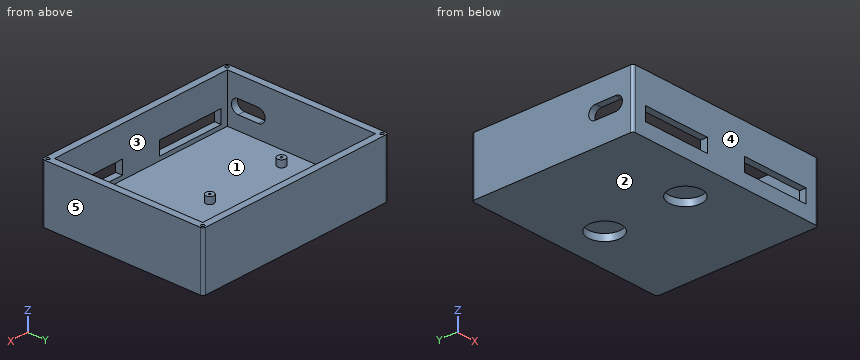
Autodesk Fusion 360 part; units mm, degrees
sketch "スケッチ6" plane through (0, 0, 0) normal (0, 0, 1) x (1, 0, 0)
  line L0 (75, -45) -> (-75, -45)
  line L1 (-75, -45) -> (-75, 75)
  line L2 (-75, 75) -> (75, 75)
  line L3 (75, 75) -> (75, -45)
  line L4 (-200, 0) -> (160, 0)
  dimension "d22" = 150
  dimension "d110" = 75
  dimension "d111" = 45
extrude "押し出し4" add sketch "スケッチ6" along normal blind 42
sketch "スケッチ7" plane through (0, 0, 42) normal (0, 0, 1) x (-1, 0, 0)
  line L0 (-75, -75) -> (75, -75)
  line L1 (75, -75) -> (75, 45)
  line L2 (75, 45) -> (-75, 45)
  line L3 (-75, 45) -> (-75, -75)
  line L4 (70, -70) -> (-70, -70)
  line L5 (-70, -70) -> (-70, 40)
  line L6 (-70, 40) -> (70, 40)
  line L7 (70, 40) -> (70, -70)
  dimension "d26" = 5
  dimension "d27" = 5
extrude "押し出し5" cut sketch "スケッチ7" against normal blind 35 contours L4 L5 L6 L7
sketch "スケッチ8" plane through (0, 0, 7) normal (0, 0, 1) x (-1, 0, 0)
  line L0 (70, 40) -> (-70, 40)
  line L1 (-70, 40) -> (-70, -70)
  line L2 (-70, -70) -> (70, -70)
  line L3 (70, -70) -> (70, 40)
  circle A0 centre (56.5, -61.5) radius 3
  circle A1 centre (-1.5, -61.5) radius 3
  circle A2 centre (56.5, -12.5) radius 3
  circle A3 centre (-1.5, -12.5) radius 3
  dimension "d32" = 6
  dimension "d35" = 6
  dimension "d37" = 58
  dimension "d41" = 6
  dimension "d42" = 6
extrude "押し出し6" add sketch "スケッチ8" along normal blind 5 contours A0 | A1 | A2 | A3
sketch "スケッチ9" plane through (0, 0, 12) normal (0, 0, 1) x (-1, 0, 0)
  circle A0 centre (56.5, -61.5) radius 3
  line L0 (56.5, -61.5) -> (53.5, -61.5)
  line L1 (56.5, -61.5) -> (56.5, -64.5)
hole "穴1" at (-56.5, 61.5, 12) direction (0, 0, -1) diameter 1.623 depth 10 tip angle 118
sketch "スケッチ10" plane through (0, 0, 12) normal (0, 0, 1) x (-1, 0, 0)
  circle A0 centre (-1.5, -61.5) radius 3
  line L0 (-1.5, -61.5) -> (-3.2909, -61.5)
  line L1 (-3.2909, -61.5) -> (-1.5, -61.5)
  line L2 (-1.5, -61.5) -> (-1.5, -64)
hole "穴2" at (1.5, 61.5, 12) direction (0, 0, -1) diameter 1.623 depth 10 tip angle 118
sketch "スケッチ11" plane through (0, 0, 12) normal (0, 0, 1) x (-1, 0, 0)
  circle A0 centre (-1.5, -12.5) radius 3
  line L0 (-1.5, -12.5) -> (-4.5, -12.5)
  line L1 (-1.5, -12.5) -> (-1.5, -15.5)
hole "穴3" at (1.5, 12.5, 12) direction (0, 0, -1) diameter 1.623 depth 10 tip angle 118
sketch "スケッチ12" plane through (0, 0, 12) normal (0, 0, 1) x (-1, 0, 0)
  circle A0 centre (56.5, -12.5) radius 3
  line L0 (56.5, -12.5) -> (53.5, -12.5)
  line L1 (56.5, -12.5) -> (56.5, -15.5)
hole "穴4" at (-56.5, 12.5, 12) direction (0, 0, -1) diameter 1.623 depth 10 tip angle 118
sketch "スケッチ13" plane through (-75, 0, 0) normal (-1, 0, 0) x (0, -1, 0)
  line L0 (-75, 0) -> (45, 0)
  line L1 (45, 0) -> (45, 42)
  line L2 (45, 42) -> (-75, 42)
  line L3 (-75, 42) -> (-75, 0)
  line L4 (17, 27) -> (32, 27)
  line L5 (32, 17) -> (25.3423, 17)
  arc A0 (32, 17) -> (32, 27) centre (32, 22) ccw
  line L6 (25.3423, 17) -> (17, 17)
  arc A1 (17, 27) -> (17, 17) centre (17, 22) ccw
  dimension "d55" = 15
  dimension "d56" = 10
extrude "押し出し7" cut sketch "スケッチ13" against normal blind 10 contours L4 L5 A0 L6 A1
sketch "スケッチ15" plane through (0, -45, 0) normal (0, -1, 0) x (1, 0, 0)
  line L0 (-75, 0) -> (75, 0)
  line L1 (75, 0) -> (75, 42)
  line L2 (75, 42) -> (-75, 42)
  line L3 (-75, 42) -> (-75, 0)
  line L4 (-15, 10) -> (-65, 10)
  line L5 (-65, 10) -> (-65, 20)
  line L6 (-65, 20) -> (-15, 20)
  line L7 (-15, 20) -> (-15, 10)
  line L8 (15, 20) -> (65, 20)
  line L9 (65, 20) -> (65, 10)
  line L10 (65, 10) -> (15, 10)
  line L11 (15, 10) -> (15, 20)
extrude "押し出し8" cut sketch "スケッチ15" against normal blind 5 contours L4 L5 L6 L7 | L8 L9 L10 L11
sketch "スケッチ16" plane through (0, 0, 42) normal (0, 0, 1) x (-1, 0, 0)
  line L0 (-70, -70) -> (-70, 40)
  line L1 (-70, 40) -> (70, 40)
  line L2 (70, 40) -> (70, -70)
  line L3 (70, -70) -> (-70, -70)
  line L4 (-75, -75) -> (75, -75)
  line L5 (75, -75) -> (75, 45)
  line L6 (75, 45) -> (-75, 45)
  line L7 (-75, 45) -> (-75, -75)
  circle A0 centre (72.5, -72.5) radius 1.5
  circle A1 centre (-72.5, -72.5) radius 1.5
  circle A2 centre (72.5, 72.5) radius 1.5
  circle A3 centre (-72.5, 72.5) radius 1.5
  dimension "d96" = 3
  dimension "d97" = 2.5
  dimension "d98" = 2.5
hole "穴5" at (-72.5, 72.5, 42) at (-72.5, -72.5, 42) at (72.5, 72.5, 42) at (72.5, -72.5, 42) direction (0, 0, -1) diameter 2.529 depth 10 tip angle 118
sketch "スケッチ17" plane through (0, 0, 0) normal (0, 0, 1) x (1, 0, 0)
  circle A0 centre (0, 45) radius 11.95
  circle A1 centre (0, -15) radius 11.95
  line L0 (-75, 75) -> (75, 75)
  line L1 (75, -45) -> (-75, -45)
  dimension "d102" = 23.9
  dimension "d103" = 23.9
  dimension "d104" = 30
  dimension "d105" = 30
extrude "押し出し9" cut sketch "スケッチ17" along normal blind 5
fillet "フィレット1" radius 2 4 edges at (75, -45, 21) (-75, -45, 21) (75, 75, 21) (-75, 75, 21)
sketch "スケッチ18" plane through (0, 0, 42) normal (0, 0, 1) x (-1, 0, 0)
  arc A0 (73, -75) -> (75, -73) centre (73, -73) ccw
  line L0 (75, -73) -> (75, 43)
  arc A1 (75, 43) -> (73, 45) centre (73, 43) ccw
  line L1 (73, 45) -> (-73, 45)
  arc A2 (-73, 45) -> (-75, 43) centre (-73, 43) ccw
  line L2 (-75, 43) -> (-75, -73)
  arc A3 (-75, -73) -> (-73, -75) centre (-73, -73) ccw
  line L3 (-73, -75) -> (73, -75)
  circle A4 centre (-72.5, -72.5) radius 1.2645
  circle A5 centre (72.5, -72.5) radius 1.2645
  line L4 (-70, -70) -> (-70, 40)
  line L5 (-70, 40) -> (70, 40)
  line L6 (70, 40) -> (70, -70)
  line L7 (70, -70) -> (-70, -70)
  circle A6 centre (72.5, 42.5) radius 1
  circle A7 centre (-72.5, 42.5) radius 1
  dimension "d112" = 2
  dimension "d113" = 2.5
  dimension "d114" = 2.5
  dimension "d115" = 2
  dimension "d116" = 2.5
  dimension "d117" = 2.5
hole "穴6" at (-72.5, -42.5, 42) at (72.5, -42.5, 42) direction (0, 0, -1) diameter 2.529 depth 10 tip angle 118
equation "d111 = 75 mm - 30 mm"
Could you check a few things on this model? Use its own coordinates, in mm. Face numbers are marked on the shaded views. A direction names the side the tool comes from. Coordinates: 2 decimals unless noted, no trailing zeros. Loops run counter-clockwise (first coordinate to the right, second up) from the corner with the lowest first, then second, coordinate; pieces in that order, holes last. Notation, with made-up numbers: (62.5, 87) -> (86.5, 87) arc R17 ccw to (86.5, 106) -> close; hole circle Ø4 at (87, 66.25). An arc over 180 degrees is marked (long way). Answer in a Markdown table with one row per item.
(1) Thinking about a two-plate mould opening in Y: for the marked faces 3, 4 and 5, which applies, released by +Y, released by -Y, zero draft, split by the parting line, or undercut?
Results found:
| item | result |
|---|---|
| face 3 | undercut |
| face 4 | released by -Y |
| face 5 | zero draft |
(2) Imagine slicing it at D-D (y = -20). List the corners of the cut face in (x, z) for me, plus the area to 3 significant figures.
Results found:
| item | result |
|---|---|
| outline | (-75, 0) -> (-10.85, 0) -> (-10.85, 5) -> (10.85, 5) -> (10.85, 0) -> (75, 0) -> (75, 42) -> (70, 42) -> (70, 7) -> (-70, 7) -> (-70, 17) -> (-75, 17) -> close; (-75, 27) -> (-70, 27) -> (-70, 42) -> (-75, 42) -> close |
| area | 1,240 mm^2 |
(3) For the marked faces 1 and 2, which set-ups out of +Z, -Z, +X, -X, +Y, -Y let a thin tool reach every point of the face, with its end or its side?
Results found:
| item | result |
|---|---|
| face 1 | +Z |
| face 2 | -Z, +X, -X, +Y, -Y |
(4) Imagine slicing it at C-C (z = 22). List the corners of the cut face in (x, y) for me.
Results found:
| item | result |
|---|---|
| outline | (-75, -43) arc R2 ccw to (-73, -45) -> (73, -45) arc R2 ccw to (75, -43) -> (75, 73) arc R2 ccw to (73, 75) -> (-73, 75) arc R2 ccw to (-75, 73) -> (-75, -12) -> (-70, -12) -> (-70, 70) -> (70, 70) -> (70, -40) -> (-70, -40) -> (-70, -37) -> (-75, -37) -> close |
(5) Imagine slicing it at B-B (y = 23). List the corners of the cut face in (x, z) for me, plus the area to 3 significant figures.
Results found:
| item | result |
|---|---|
| outline | (-75, 0) -> (75, 0) -> (75, 42) -> (70, 42) -> (70, 7) -> (-70, 7) -> (-70, 42) -> (-75, 42) -> close |
| area | 1,400 mm^2 |
(6) Will these pins go through, and if not, where does the flat tip stop? pin 1 Ø1 at (x, y) = (-42.5, 39.5) entering from +Z; pin 2 Ø2 at (x, y) = (1.5, 61.5) entering from +Z; pin 3 Ø1 at (x, y) = (0, -9) entering from -Z.
Results found:
| item | result |
|---|---|
| pin 1 | stops at z = 7 |
| pin 2 | stops at z = 12 |
| pin 3 | stops at z = 5 |
(7) Imagine slicing it at A-A (x = -25). List the corners of the cut face in (y, z) for me, plus the area to 3 significant figures.
Results found:
| item | result |
|---|---|
| outline | (-45, 0) -> (75, 0) -> (75, 42) -> (70, 42) -> (70, 7) -> (-40, 7) -> (-40, 10) -> (-45, 10) -> close; (-45, 20) -> (-40, 20) -> (-40, 42) -> (-45, 42) -> close |
| area | 1,140 mm^2 |
(8) If I drill on probe 1 along Y at (x, z) = (0, 1.3); probe 2 along Y at (x, z) = (-72.5, 35); probe 3 along X at (y, z) = (-42.5, 37.75), over which ranges is the centre line in solid material (lowest first)?
Results found:
| item | result |
|---|---|
| probe 1 | y = -45 to -26.95, -3.05 to 33.05, 56.95 to 75 |
| probe 2 | y = -45 to -43.76, -41.24 to 71.24, 73.76 to 75 |
| probe 3 | x = -75 to -73.76, -71.24 to 71.24, 73.76 to 75 |
